from build123d import *

# Parameters (mm, degrees)
SKETCH_1_R          = 34
SKETCH_1_R_2        = 2.05
SKETCH_1_R_3        = 6
EXTRUDE_1_DEPTH     = 4
SKETCH_5_R          = 6.5
SKETCH_5_R_2        = 5
EXTRUDE_4_DEPTH     = 1.5
EXTRUDE_START       = 2
SKETCH_6_R          = 7
SKETCH_6_R_2        = 6
EXTRUDE_5_DEPTH     = 2
EXTRUDE_START_2     = -4
EXTRUDE_6_DEPTH     = 4
SKETCH_9_R          = 2.25
SKETCH_9_R_2        = 3.05
CUT_EXTRUDE_1_DEPTH = 10
CHAMFER_2_SIZE      = 3.6
SKETCH_10_R         = 6.05
CUT_EXTRUDE_3_DEPTH = 4.5


with BuildPart() as part:
    # 草图1 → 凸台-拉伸1 (new body)
    with BuildSketch(Plane(origin=(0, 0, 0), x_dir=(1, 0, 0), z_dir=(0, 1, 0))):
        with Locations(Location((0, 0, 0), (0, 0, 270))):
            Circle(SKETCH_1_R)
        with Locations(Location((0, 14, 0), (0, 0, 270))):
            Circle(SKETCH_1_R_2, mode=Mode.SUBTRACT)
        with Locations(Location((12.124355653, 7, 0), (0, 0, 270))):
            Circle(SKETCH_1_R_2, mode=Mode.SUBTRACT)
        with Locations(Location((12.124355653, -7, 0), (0, 0, 270))):
            Circle(SKETCH_1_R_2, mode=Mode.SUBTRACT)
        with Locations(Location((0, -14, 0), (0, 0, 270))):
            Circle(SKETCH_1_R_2, mode=Mode.SUBTRACT)
        with Locations(Location((-12.124355653, -7, 0), (0, 0, 270))):
            Circle(SKETCH_1_R_2, mode=Mode.SUBTRACT)
        with Locations(Location((-12.124355653, 7, 0), (0, 0, 270))):
            Circle(SKETCH_1_R_2, mode=Mode.SUBTRACT)
        with Locations(Location((0, 0, 0), (0, 0, 270))):
            Circle(SKETCH_1_R_3, mode=Mode.SUBTRACT)
    extrude(amount=EXTRUDE_1_DEPTH)

    # 草图5 → 凸台-拉伸4 (add)
    with BuildSketch(Plane(origin=(0, 4, 0), x_dir=(1, 0, 0), z_dir=(0, 1, 0))):
        Circle(SKETCH_5_R)
        with Locations(Location((0, 0, 0), (0, 0, 270))):
            Circle(SKETCH_5_R_2, mode=Mode.SUBTRACT)
    extrude(amount=-EXTRUDE_4_DEPTH)

    # 草图6 → 凸台-拉伸5 (add)
    with BuildSketch(Plane(origin=(0, 0, 0), x_dir=(-1, 0, 0), z_dir=(0, -1, 0)).offset(EXTRUDE_START)):
        with Locations(Location((0, 0, 0), (0, 0, 270))):
            Circle(SKETCH_6_R)
        with Locations(Location((0, 0, 0), (0, 0, 90))):
            Circle(SKETCH_6_R_2, mode=Mode.SUBTRACT)
    extrude(amount=-EXTRUDE_5_DEPTH)

    # 草图8 → 凸台-拉伸6 (add)
    with BuildSketch(Plane(origin=(0, 4, 0), x_dir=(1, 0, 0), z_dir=(0, 1, 0)).offset(EXTRUDE_START_2)):
        with BuildLine():
            Line((-8.707638575, -46.70307303), (51.809561134, -11.522559398))
            Line((51.809561134, -11.522559398), (15.62388997, 50.723703159))
            Line((15.62388997, 50.723703159), (-44.893309739, 15.543189527))
            Line((-44.893309739, 15.543189527), (-33.818604688, -3.507417415))
            ThreePointArc((-33.818604688, -3.507417415), (-1.756052475, 33.954620889), (34, 0))
            ThreePointArc((34, 0), (15.546708924, -30.237391449), (-19.782343625, -27.652466087))
            Line((-19.782343625, -27.652466087), (-8.707638575, -46.70307303))
        make_face()
    extrude(amount=EXTRUDE_6_DEPTH)

    # 草图9 → 切除-拉伸1 (cut)
    with BuildSketch(Plane(origin=(0, 0, 0), x_dir=(-1, 0, 0), z_dir=(0, -1, 0))):
        with Locations(Location((-36.730998817, -10.456276868, 0), (0, 0, 90))):
            Circle(SKETCH_9_R)
        with Locations(Location((-9.089166677, 37.092951475, 0), (0, 0, 90))):
            Circle(SKETCH_9_R)
        with Locations(Location((-17.279041767, -21.764299107, 0), (0, 0, 90))):
            Circle(SKETCH_9_R_2)
        with Locations(Location((2.172915282, -33.072321345, 0), (0, 0, 90))):
            Circle(SKETCH_9_R)
        with Locations(Location((29.814747421, 14.476906997, 0), (0, 0, 90))):
            Circle(SKETCH_9_R)
        with Locations(Location((10.362790372, 25.784929236, 0), (0, 0, 90))):
            Circle(SKETCH_9_R_2)
    extrude(amount=-CUT_EXTRUDE_1_DEPTH, mode=Mode.SUBTRACT)

    # 倒角2
    chamfer_2_edges = [part.edges().sort_by_distance(p)[0] for p in [
        (17.279041767, 4, 24.814299107),
        (-10.362790372, 4, -22.734929236),
    ]]
    chamfer(chamfer_2_edges, length=CHAMFER_2_SIZE)

    # 草图10 → 切除-拉伸3 (cut)
    with BuildSketch(Plane(origin=(0, -2, 0), x_dir=(-1, 0, 0), z_dir=(0, -1, 0))):
        with Locations(Location((0, 0, 0), (0, 0, 90))):
            Circle(SKETCH_10_R)
    extrude(amount=-CUT_EXTRUDE_3_DEPTH, mode=Mode.SUBTRACT)


solid = part.part
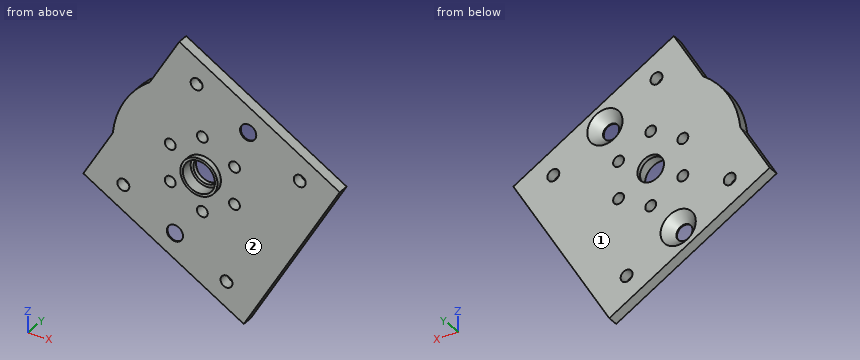
Verification items for the finished model (mm, model axes). Face numbers are marked on the shaded views. Round coordinates to 2 decimals unless told otherwise and drop trailing zeros. Loops run counter-clockwise (first coordinate to the right, second up) from the corner with the lowest first, then second, coordinate; pieces in that order, holes last. Notation, with made-up numbers: (19, -23.75) - (76, -23.75) arc R11 cw to (76, -4.75) - close; hole circle Ø7 at (-31, -30). An arc over 180 degrees is marked (long way). Use one line per item in the form item = value.
1. Draft check along Y on the marked faces 1 and 2. Enter one of: pulls with the +Y half, pulls with the -Y half, needs draft (parallel to the pull), parting line crosses it, or undercut.
A:
face_1 = pulls with the +Y half
face_2 = pulls with the -Y half
2. Section check D-D on z = 0. Record the cut outline in (x, y).
A:
outline = (-35.86, 0) - (-7, 0) - (-7, -2) - (-6.05, -2) - (-6.05, 2.5) - (-5, 2.5) - (-5, 4) - (-35.86, 4) - close; (5, 2.5) - (6.05, 2.5) - (6.05, -2) - (7, -2) - (7, 0) - (45.11, 0) - (45.11, 4) - (5, 4) - close
3. Scan lines: probe 1 along X at (y, z) = (-0.1, 0); probe 2 along X at (y, z) = (2.05, 7); probe 3 along X at (y, z) = (3, -7). Record each from-to range of solid material in increasing order.
A:
probe_1 = -7 to -6.05, 6.05 to 7
probe_2 = -33.27 to -14.17, -10.07 to 10.07, 14.17 to 49.18
probe_3 = -39.93 to -14.17, -10.07 to 10.07, 14.17 to 41.04
4. Section check A-A on z = 14. Record the cut outline in (x, y).
A:
outline = (-30.98, 0) - (-2.05, 0) - (-2.05, 4) - (-30.98, 4) - close; (2.05, 0) - (47.55, 0) - (47.55, 4) - (2.05, 4) - close
5. Gauge pin test, flat ends, axial feed: pin 1 Ø8 at (x, z) = (-10.36, -25.78) entering from +Y; pin 2 Ø6.5 at (x, z) = (0, -14) entering from -Y; pin 3 Ø3 at (x, y) = (-15.5, 0.5) entering from +Z. Record the tip position at first contact, or that the pin passes through.
A:
pin_1 = 1.36
pin_2 = 0
pin_3 = 37.6
6. Section check B-B on z = -14. Record the cut outline in (x, y).
A:
outline = (-44, 0) - (-32.01, 0) - (-32.01, 4) - (-44, 4) - close; (-27.62, 0) - (-2.05, 0) - (-2.05, 4) - (-27.62, 4) - close; (2.05, 0) - (36.97, 0) - (36.97, 4) - (2.05, 4) - close
7. Section check C-C on y = 1.55. Give the number of separate pieces and of enclosed holes in the cut face, and give its area (3 significant figures).
A:
separate_pieces = 1
enclosed_holes = 13
area = 4,730 mm²
